```python
from build123d import *

# Parameters (mm, degrees)
WISHBONE_END_BASE_BODY_DEPTH           = 6.35
WISHBONE_END_BASE_BODY_DEPTH_BACK      = 6.35
WISHBONE_END_BODY_SKETCH_R             = 7.6199999999999655
SPHERICAL_BEARING_BORE_HOLE_DEPTH      = 994.1778562213065
SPHERICAL_BEARING_BORE_HOLE_DEPTH_BACK = 3.2385
SKETCH37_R                             = 9.398000000000074
GROOVE_START                           = 3.2385
SKETCH38_R                             = 10.10920000000004
GROOVE_FOR_99142A390_DEPTH             = 0.9905999999999999
SKETCH39_R                             = 6.172199999999972
LEADING_ARM_TUBE_INSERT_DEPTH          = 15.875
SKETCH40_R                             = 6.172199999999972
TRAILING_ARM_TUBE_INSERT_DEPTH         = 15.875
CUT_EXTRUDE3_DEPTH                     = 614.178901904527
CUT_EXTRUDE3_DEPTH_BACK                = 614.178901904527
FILLET1_R                              = 9.525
CHAMFER1_SIZE                          = 3.8099999999999996
FILLET2_R                              = 9.525
FILLET3_R                              = 1.5875
SKETCH42_R                             = 1.587499999999916
SKETCH42_R_2                           = 1.5874999999997772
SKETCH42_R_3                           = 1.5875000000002346
MACHINING_ALIGNMENT_HOLES_DEPTH        = 993.6874865506448


with BuildPart() as part:
    # wishbone end body sketch → wishbone end base body (new, two sides: drawn at the far end of the back side and taken through both)
    with BuildSketch(Plane(origin=(0.7258862866452951, 134.87955098448836, 3.3083663449025464), x_dir=(0.999985527474362, -0.005378423373816958, -0.00013192359218796315), z_dir=(0.005380041061385716, 0.9996848486991856, 0.024520571760546048)).offset(-WISHBONE_END_BASE_BODY_DEPTH_BACK)):
        with BuildLine():
            Line((-590.7162762655777, -779.9030929511134), (-558.8429156016132, -791.9248886865561))
            Line((-558.8429156016132, -791.9248886865561), (-549.8791042276648, -768.1591552526331))
            Line((-549.8791042276648, -768.1591552526331), (-558.6610183956265, -744.3256078132241))
            Line((-558.6610183956265, -744.3256078132241), (-590.6253276625844, -756.1034525144474))
            ThreePointArc((-590.6253276625844, -756.1034525144474), (-598.9342778486073, -767.9716944579083), (-590.7162762655777, -779.9030929511134))
        make_face()
        with Locations(Location((-586.2343705786035, -768.0202262341521, 0), (0, 0, 270))):
            Circle(WISHBONE_END_BODY_SKETCH_R, mode=Mode.SUBTRACT)
    extrude(amount=WISHBONE_END_BASE_BODY_DEPTH + WISHBONE_END_BASE_BODY_DEPTH_BACK)

    # Sketch37 → spherical bearing bore hole (cut, two sides: drawn at the far end of the back side and taken through both)
    with BuildSketch(Plane(origin=(0.7258862866452951, 134.87955098448836, 3.3083663449025464), x_dir=(0.999985527474362, -0.005378423373816958, -0.00013192359218796315), z_dir=(0.005380041061385716, 0.9996848486991856, 0.024520571760546048)).offset(-SPHERICAL_BEARING_BORE_HOLE_DEPTH_BACK)):
        with Locations(Location((-586.2343705786035, -768.0202262341521, 0), (0, 0, 270))):
            Circle(SKETCH37_R)
    extrude(amount=SPHERICAL_BEARING_BORE_HOLE_DEPTH + SPHERICAL_BEARING_BORE_HOLE_DEPTH_BACK, mode=Mode.SUBTRACT)

    # Sketch38 → groove for 99142A390 (cut)
    with BuildSketch(Plane(origin=(0.7258862866452951, 134.87955098448836, 3.3083663449025464), x_dir=(0.999985527474362, -0.005378423373816958, -0.00013192359218796315), z_dir=(0.005380041061385716, 0.9996848486991856, 0.024520571760546048)).offset(GROOVE_START)):
        with Locations(Location((-586.2343705786035, -768.0202262341521, 0), (0, 0, 270))):
            Circle(SKETCH38_R)
    extrude(amount=-GROOVE_FOR_99142A390_DEPTH, mode=Mode.SUBTRACT)

    # Sketch39 → leading arm tube insert (add)
    with BuildSketch(Plane(origin=(-227.74660652476513, 3.3313146383369725, -85.84541568022186), x_dir=(0.3526386884421761, -0.005158146778901092, -0.9357453440630037), z_dir=(0.9356452552652121, -0.013685950287986396, 0.3526764112673413))):
        with Locations(Location((-928.7082188867262, 110.62389056036547, 0), (0, 0, 0.295569033))):
            Circle(SKETCH39_R)
    extrude(amount=LEADING_ARM_TUBE_INSERT_DEPTH)

    # Sketch40 → trailing arm tube insert (add)
    with BuildSketch(Plane(origin=(-733.3441053167152, -2.681708402002071, 270.23369281713326), x_dir=(-0.3457621685662157, -0.0012643904898342719, -0.938321333075763), z_dir=(0.9383150593615196, 0.003431250568691938, -0.34576448038357405))):
        with Locations(Location((-521.3169196855705, 121.34025761798294, 0), (0, 0, 0.072444684))):
            Circle(SKETCH40_R)
    extrude(amount=TRAILING_ARM_TUBE_INSERT_DEPTH)

    # Sketch41 → Cut-Extrude3 (cut, two sides: drawn at the far end of the back side and taken through both)
    with BuildSketch(Plane(origin=(-2.943409073321915, -18.871393740527775, 770.0180176181074), x_dir=(-0.9999926986368375, 9.362436458525497e-05, -0.003820197310804283), z_dir=(0.0038213443989151604, 0.024500194493421494, -0.9996925216269098)).offset(-CUT_EXTRUDE3_DEPTH_BACK)):
        Polygon((595.2948241213879, 131.77671300237452), (595.2873859667309, 133.15922897461502), (557.1948241213879, 133.159228974615), (557.1948241213879, 131.571728974615), align=None)
        Polygon((595.2350378549631, 142.88907514922224), (557.126497101028, 142.68404517085534), (557.126497101028, 144.27154517085532), (595.226497101028, 144.47652919861486), align=None)
    extrude(amount=CUT_EXTRUDE3_DEPTH + CUT_EXTRUDE3_DEPTH_BACK, mode=Mode.SUBTRACT)

    # Fillet1
    # the kernel refuses this fillet: 9.525 mm, written as the material it adds along each edge
    with BuildSketch(Plane(origin=(-560.2724336268298, 113.41353360474875, 807.3240128802753), x_dir=(-3.2942809255927247e-12, -0.9996998207983545, -0.02450037337955774), z_dir=(0.0038213443989151483, 0.024500194493421494, -0.9996925216269098))) as fillet1_piece_1_section:
        with BuildLine():
            CenterArc((9.525000000017343, 5.265141854675068), FILLET1_R, 179.99999999981125, 33.55730976200755)
            Line((1.734599e-11, 5.265141854706447), (-0.19049999998265063, 5.265141854707075))
            Line((-0.19049999998265063, 5.265141854707075), (-0.1904999999999994, 6.2734e-13))
            Line((-0.1904999999999994, 6.2734e-13), (-6.2619e-13, -0.19050000000003728))
            ThreePointArc((-6.2619e-13, -0.19050000000003728), (0.7937500000033896, -0.19050000000265227), (1.4287500000078057, -0.10530283709351278))
            Line((1.4287500000078057, -0.10530283709351278), (1.5875000000079915, 0))
        make_face()
    fillet1_piece_1 = extrude(amount=72.36652834652159, mode=Mode.PRIVATE)
    fillet1_piece_1 = split(fillet1_piece_1, bisect_by=Plane(origin=(-569.064048669562, 113.51391058502266, 790.8244812436348), z_dir=(0.35290085216371403, 0.021045143050144578, -0.9354240164204272)), keep=Keep.TOP, mode=Mode.PRIVATE)
    fillet1_piece_1 = split(fillet1_piece_1, bisect_by=Plane(origin=(-568.9133352872509, 114.4801954294582, 751.396723516925), z_dir=(0.34573964848360106, -0.024868248849107495, 0.9380008878810375)), keep=Keep.TOP, mode=Mode.PRIVATE)
    add(fillet1_piece_1)
    with BuildSketch(Plane(origin=(-559.9274640787987, 124.70915530829745, 735.1857328131279), x_dir=(-0.9999782260055279, 0.005472088364658121, -0.0036883280448706773), z_dir=(-0.0038213443989151483, -0.024500194493421494, 0.9996925216269098))) as fillet1_piece_2_section:
        with BuildLine():
            CenterArc((5.273648095245833, -9.525000000000006), FILLET1_R, 89.99999999999999, 33.55705973982701)
            Line((0.00854087754486855, -1.5874770245300465), (-0.09676126680913032, -1.4287265650206478))
            ThreePointArc((-0.09676126680913032, -1.4287265650206478), (-0.18622680417126483, -0.794763417570426), (-0.19049724294364254, -0.0010249053053967))
            Line((-0.19049724294364254, -0.0010249053053967), (-2.955e-14, 0.19049999999999728))
            Line((-2.955e-14, 0.19049999999999728), (5.2736480952458065, 0.1904999999999973))
            Line((5.2736480952458065, 0.1904999999999973), (5.273648095245836, 0))
        make_face()
    fillet1_piece_2 = extrude(amount=72.42179621801027, mode=Mode.PRIVATE)
    fillet1_piece_2 = split(fillet1_piece_2, bisect_by=Plane(origin=(-569.0001389759076, 123.73065535763696, 791.0784480398987), z_dir=(0.35290085216371403, 0.021045143050144578, -0.9354240164204272)), keep=Keep.TOP, mode=Mode.PRIVATE)
    fillet1_piece_2 = split(fillet1_piece_2, bisect_by=Plane(origin=(-568.8494001928565, 124.697103483473, 751.6440278829348), z_dir=(0.34573964848360106, -0.024868248849107495, 0.9380008878810375)), keep=Keep.TOP, mode=Mode.PRIVATE)
    add(fillet1_piece_2)

    # Chamfer1
    chamfer1_edges = [part.edges().sort_by_distance(p)[0] for p in [
        (-558.1089414465442, 118.46651268395277, 795.0688611446163),
        (-557.9270468730695, 119.63271283819378, 747.4838685753589),
    ]]
    chamfer(chamfer1_edges, length=CHAMFER1_SIZE)

    # Fillet2
    fillet2_edges = [part.edges().sort_by_distance(p)[0] for p in [
        (-549.1452598015858, 119.00105931742645, 771.3090911275373),
    ]]
    fillet(fillet2_edges, radius=FILLET2_R)

    # Fillet3
    fillet3_edges = [part.edges().sort_by_distance(p)[0] for p in [
        (-561.5020537397296, 119.61471747963421, 748.801110510107),
        (-561.6737763595983, 118.51373386067205, 793.7250432821822),
        (-556.764389199803, 118.54669467897371, 791.5048956420608),
        (-556.6097788123484, 119.53796481007879, 751.0576519581815),
    ]]
    fillet(fillet3_edges, radius=FILLET3_R)

    # Sketch42 → machining alignment holes (cut, through all)
    with BuildSketch(Plane(origin=(0.7515088558077796, 139.6405730446522, 3.42514613128373), x_dir=(0.9999855274743621, -0.005378423373807206, -0.0001319235921877165), z_dir=(0.005380041061375963, 0.9996848486991857, 0.024520571760544684))):
        with Locations(Location((-568.57694591022, -761.514019457373, 0), (0, 0, 270))):
            Circle(SKETCH42_R)
        with Locations(Location((-568.6271868865741, -774.6611941588587, 0), (0, 0, 270))):
            Circle(SKETCH42_R)
        with Locations(Location((-572.9243944265849, -773.0404001728256, 0), (0, 0, 270))):
            Circle(SKETCH42_R_2)
        with Locations(Location((-572.8864152580355, -763.1019236507452, 0), (0, 0, 270))):
            Circle(SKETCH42_R_3)
    extrude(amount=-MACHINING_ALIGNMENT_HOLES_DEPTH, mode=Mode.SUBTRACT)


solid = part.part
```
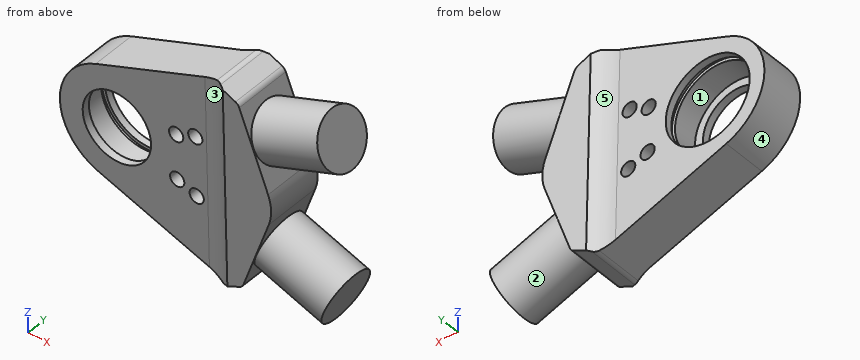
Source: CAD feature listing. Evaluate the final solid. Frame: model axes, mm. Face numbers are marked on the shaded views. A direction names the side the tool comes from. Coordinates: 2 decimals unless noted, no trailing zeros. Put each result on its own line as item: value. Start each with the question number.
1) Ray query, L1, parallel to X at y = 119.75, z = 776; L2, parallel to X at y = 120.75, z = 765.5; L3, parallel to X at y = 118, z = 772. Return the intervals inside material, ascending. Write a range as from..to.
2) Contact query for flat-ended pins moving along their axis: pin 1 Ø8 at (y, z) = (122, 776.5) entering from -X; pin 2 Ø3 at (x, z) = (-589, 780.5) entering from -Y; pin 3 Ø2 at (y, z) = (119, 768.5) entering from +X. Output: stop coordinate, or through.
3) Cut plane A-A on x = -567. Give the number of separate pieces and of enclosed holes in the cut face, then the cut area to 3 significant figures.
4) Pull-direction query (Y, two-part tool) for the marked faces 1, 2 and 3; classes: pulls with the +Y half, pulls with the -Y half, needs draft (parallel to the pull), parting line crosses it, or undercut.
5) Reachability of the marked faces 4 and 5 from +Z, -Z, +X, -X, +Y, -Y: full face, straight path, thin tool, end or side. Return the list, or none.
The answers:
1. L1: x = -597.25..-593.57, -577.42..-573.76, -570.61..-550.9
1. L2: x = -596.84..-592.96, -578.03..-573.52, -570.77..-569.21, -566.46..-551.29
1. L3: x = -598.18..-594.87, -576.15..-549.82
2. pin 1: stops at x = -598.12
2. pin 2: stops at y = 114.03
2. pin 3: stops at x = -549.95
3. separate pieces: 3
3. enclosed holes: 0
3. area: 340 mm²
4. face 1: undercut
4. face 2: parting line crosses it
4. face 3: pulls with the -Y half
5. face 4: -X
5. face 5: +Z, +Y
